```python
from build123d import *

# Parameters (mm, degrees)
F1_DEPTH = 25


with BuildPart() as f1:
    # F0 (on Front) → F1 (new body)
    with BuildSketch(Plane.XZ):
        with BuildLine():
            Line((0, 15), (0, 0))
            Line((0, 0), (15, 0))
            Line((15, 0), (24, 20))
            Line((24, 20), (100, 20))
            Line((100, 20), (110, 0))
            Line((110, 0), (135, 0))
            Line((135, 0), (125, 20))
            Line((125, 20), (143.143047, 12.742781))
            ThreePointArc((143.143047, 12.742781), (147.803144, 13.244829), (150, 17.385165))
            Line((150, 17.385165), (150, 77.679492))
            ThreePointArc((150, 77.679492), (145, 86.339746), (135, 86.339746))
            Line((135, 86.339746), (115.358984, 75))
            Line((115.358984, 75), (90, 75))
            Line((90, 75), (90, 95))
            Line((90, 95), (79.641016, 95))
            ThreePointArc((79.641016, 95), (45, 75), (10.358984, 95))
            Line((10.358984, 95), (0, 95))
            Line((0, 95), (0, 75))
            Line((0, 75), (30, 45))
            Line((30, 45), (10, 45))
            Line((10, 45), (0, 15))
        make_face()
        with BuildLine():
            ThreePointArc((60.976671, 30.642377), (44.221825, 29.221825), (45.642377, 45.976671))
            Line((45.642377, 45.976671), (69.532205, 62.896366))
            ThreePointArc((69.532205, 62.896366), (77.242641, 62.242641), (77.896366, 54.532205))
            Line((77.896366, 54.532205), (60.976671, 30.642377))
        make_face(mode=Mode.SUBTRACT)
        Polygon((114.547005, 45), (108.773503, 35), (97.226497, 35), (91.452995, 45), (97.226497, 55), (108.773503, 55), align=None, mode=Mode.SUBTRACT)
    extrude(amount=F1_DEPTH)


solid = f1.part
```
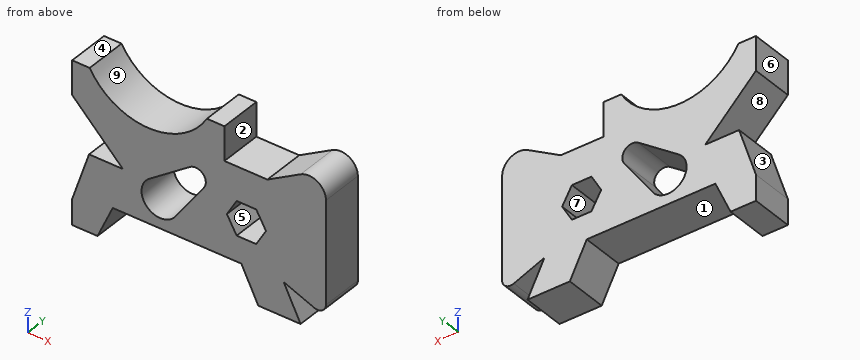
Can you work these out from the model? Positions are in its coordinate system, mm. Face numbers are marked on the shaded views. A direction names the side the tool comes from. Coordinates: 2 decimals unless noted, no trailing zeros. Order: outer loops, then holes, each group sorted by start corner. A loop starts at its lowest first (then second) coordinate and runs counter-clockwise, first axis right, second up.
1. If we section it at B-B (y = -9.5): Give the number of separate pieces and of enclosed holes in the cut face, then the cut area to 3 significant figures.
2. Thinking about a two-plate mould opening in Z: for the marked faces 6, 7, 8 and 9, which applies, +Z half, -Z half, draft (parallel to the pull), parting line (faces both ways), or undercut?
3. If we section it at C-C (z = 37): Please give me the cut outline in (x, y).
4. If we section it at A-A (x = 127): Please give me the cut outline in (y, z).
5. If we section it at D-D (x = 52): Please give me the cut outline in (y, z), then the cut area to 3 significant figures.
6. I need wall thicknesses on line 1 (X direction, y = -9.75, z = 48); line 2 (X direction, y = -8.5, z = 37); line 3 (Z direction, x = 72.5, y = -18.25). Which ranges of each line are inside material? Lowest first, please.
7. For the marked faces 1, 2, 3, 4 and 5, which set-ups out of +Z, -Z, +X, -X, +Y, -Y let a thin tool reach every point of the face, with its end or its side?
8. I'm going to push flat-ended pins straight in: pin 1 (4 mm diameter, centred on x = 55, y = -5.5, fed in from -Z); pin 2 (3 mm diameter, centred on x = 101.5, y = -6, fed in from +Z); pin 3 (13 mm diameter, centred on x = 52, z = 37, fed in from -Y); pin 4 (1 mm diameter, centred on y = -18.5, z = 58, fed in from -X). Where does each tip first touch, or does it pass through?
Entries:
1. separate pieces: 1
1. enclosed holes: 2
1. area: 8,640 mm2
2. face 6: draft
2. face 7: undercut
2. face 8: undercut
2. face 9: +Z half
3. outline: (7.33, -25) - (41, -25) - (41, 0) - (7.33, 0) - close; (65.48, -25) - (96.07, -25) - (96.07, 0) - (65.48, 0) - close; (109.93, -25) - (150, -25) - (150, 0) - (109.93, 0) - close
4. outline: (-25, 0) - (0, 0) - (0, 16) - (-25, 16) - close; (-25, 19.2) - (0, 19.2) - (0, 81.72) - (-25, 81.72) - close
5. outline: (-25, 20) - (0, 20) - (0, 26) - (-25, 26) - close; (-25, 50.48) - (0, 50.48) - (0, 75.62) - (-25, 75.62) - close
5. area: 778 mm2
6. line 1: x = 27 to 48.5, 73.27 to 93.19, 112.81 to 150
6. line 2: x = 7.33 to 41, 65.48 to 96.07, 109.93 to 150
6. line 3: z = 20 to 46.91, 63.98 to 85.95
7. face 1: -Z, +Y, -Y
7. face 2: +Z, +Y, -Y
7. face 3: -X, +Y, -Y
7. face 4: +Z, +X, -X, +Y, -Y
7. face 5: +Y, -Y
8. pin 1: stops at z = 20
8. pin 2: stops at z = 75
8. pin 3: passes through
8. pin 4: stops at x = 16.5
